Check sheet for the modelled part. Datum: model origin and axes. Units: mm. A direction names the side the tool comes from. Give positions to 0.01 mm unless a question says otherwise; leave off trailing zeros. Order: outer loops, then holes, each group sorted by start corner. A loop starts at its lowest first (then second) coordinate and runs counter-clockwise, first axis right, second up.
Autodesk Inventor part; units mm, degrees
ref_plane "YZ Plane" through (0, 0, 0) normal (1, 0, 0) x (0, 1, 0)
ref_plane "XZ Plane" through (0, 0, 0) normal (0, 1, 0) x (-1, 0, 0)
ref_plane "XY Plane" through (0, 0, 0) normal (0, 0, 1) x (1, 0, 0)
sketch "Sketch1" plane through (0, 0, 0) normal (1, 0, 0) x (0, 1, 0)
  circle A0 centre (0, 0) radius 4.7625
  dimension "d0" = 9.525
extrude "Extrusion1" add sketch "Sketch1" along normal blind 177.8
sketch "Sketch2" plane through (177.8, 0, 0) normal (1, 0, 0) x (0, 0, -1)
  circle A0 centre (0, 0) radius 4.7625
hole "Hole1" at (177.8, 0, 0) direction (-1, 0, 0) diameter 4.3434 depth 19.05 tip angle 118
sketch "Sketch3" plane through (0, 0, 0) normal (-1, 0, 0) x (0, 0, 1)
  circle A0 centre (0, 0) radius 2.1717
hole "Hole2" at (0, 0, 0) direction (1, 0, 0) diameter 4.3434 depth 19.05 tip angle 118
properties part number "STOCK,HOOD,SPACER,10-32,6.25in" material "Aluminum 6061"
Q1. Tool access check on faces 4 (the cylindrical face through (168.14, 2.12, 0.47)), 5 (the flat face through (0, 2.05, 1.13)), 6 (the cylindrical face through (9.66, 2.12, -0.47)). Record the directions out of +Z, -Z, +X, -X, +Y, -Y that give a thin tool (end or side, any length) a straight path to the whole face; none if there is none.
Q2. Sectioned sample at A-A, the plane x = 22.5. Record the cut outline in (y, z) (1 decimal), plus the area to 3 significant figures.
Q3. Material ranges on line 1 (Z direction, x = 7.5, y = 0); line 2 (Z direction, x = 165.5, y = -0.5); line 3 (Y direction, x = 98, z = 0.75), recorded low to high.
Q4. Go/stop test with flat-tipped pins: P1, Ø2, axis at x = 148.5, y = -3.5, coming from the +Z side; P2, Ø1, axis at x = 137.5, y = -2.5, coming from the -Z side; P3, Ø3, axis at x = 61, z = 4, coming from the +Y side. Record where each tip stops, or that it passes through.
Q5. Draft check along Z on faces 1 (the conical face through (157.67, 0.11, -0.36)), 2 (the flat face through (177.8, 2.05, 1.13)), 3 (the cylindrical face through (87.66, -3.78, 2.9)). Enter one of: pulls with the +Z half, pulls with the -Z half, needs draft (parallel to the pull), parting line crosses it, or undercut.
Filled in:
1. face 4: +X
1. face 5: +Z, -Z, -X, +Y, -Y
1. face 6: -X
2. outline: circle Ø9.5 at (0, 0)
2. area: 71.3 mm2
3. line 1: z = -4.76 to -2.17, 2.17 to 4.76
3. line 2: z = -4.74 to -2.11, 2.11 to 4.74
3. line 3: y = -4.7 to 4.7
4. P1: stops at z = 4.05
4. P2: stops at z = -4.32
4. P3: stops at y = 4.05
5. face 1: undercut
5. face 2: needs draft
5. face 3: parting line crosses it
